```python
from build123d import *

# Parameters (mm, degrees)
CROQUIS1_W                        = 55
CROQUIS1_H                        = 58
CROQUIS1_R                        = 2.2
SALIENTE_EXTRUIR1_DEPTH           = 6
CROQUIS2_R                        = 4.5
CORTAR_EXTRUIR1_DEPTH             = 3
REDONDEO1_R                       = 1
CROQUIS3_W                        = 55
CROQUIS3_H                        = 40
SALIENTE_EXTRUIR2_DEPTH           = 5
CROQUIS4_W                        = 55
CROQUIS4_H                        = 10
SALIENTE_EXTRUIR3_DEPTH           = 14
CORTAR_EXTRUIR2_DEPTH             = 71.577971067
CORTAR_EXTRUIR2_DEPTH_BACK        = 71.577971067
CROQUIS5_R                        = 3.3
CORTAR_EXTRUIR3_REACH             = 127.623
SALIENTE_EXTRUIR4_REACH           = 69.47
CORTAR_EXTRUIR4_DEPTH             = 118.48297749
CORTAR_EXTRUIR5_REACH             = 99.372
CORTAR_EXTRUIR5_DIRECTION_2_REACH = 99.372
CROQUIS10_W                       = 21
CROQUIS10_H                       = 42
CORTAR_EXTRUIR6_DEPTH             = 98.371710471
CROQUIS11_W                       = 33
CROQUIS11_H                       = 63.666666667
CORTAR_EXTRUIR7_DEPTH             = 5.5
CROQUIS12_R                       = 2
CORTAR_EXTRUIR8_DEPTH             = 97.106711524
CORTAR_EXTRUIR9_DEPTH             = 3
CHAFL_N1_SIZE                     = 2
CROQUIS14_R                       = 1.75
CORTAR_EXTRUIR10_DEPTH            = 98.371710471
CORTAR_EXTRUIR11_DEPTH            = 2.5
REDONDEO2_R                       = 5


with BuildPart() as part:
    # Croquis1 → Saliente-Extruir1 (new body)
    with BuildSketch(Plane(origin=(0, 0, 0), x_dir=(1, 0, 0), z_dir=(0, 1, 0))):
        Rectangle(CROQUIS1_W, CROQUIS1_H)
        with Locations(Location((-12.5, 13.181818182, 0), (0, 0, 270))):
            Circle(CROQUIS1_R, mode=Mode.SUBTRACT)
        with Locations(Location((12.5, 13.181818182, 0), (0, 0, 270))):
            Circle(CROQUIS1_R, mode=Mode.SUBTRACT)
        with Locations(Location((-12.5, -13.181818182, 0), (0, 0, 270))):
            Circle(CROQUIS1_R, mode=Mode.SUBTRACT)
        with Locations(Location((12.5, -13.181818182, 0), (0, 0, 270))):
            Circle(CROQUIS1_R, mode=Mode.SUBTRACT)
    extrude(amount=SALIENTE_EXTRUIR1_DEPTH)

    # Croquis2 → Cortar-Extruir1 (cut)
    with BuildSketch(Plane(origin=(0, 6, 0), x_dir=(1, 0, 0), z_dir=(0, 1, 0))):
        with Locations(Location((-12.5, 13.181818182, 0), (0, 0, 270))):
            Circle(CROQUIS2_R)
        with Locations(Location((12.5, 13.181818182, 0), (0, 0, 270))):
            Circle(CROQUIS2_R)
        with Locations(Location((-12.5, -13.181818182, 0), (0, 0, 270))):
            Circle(CROQUIS2_R)
        with Locations(Location((12.5, -13.181818182, 0), (0, 0, 270))):
            Circle(CROQUIS2_R)
    extrude(amount=-CORTAR_EXTRUIR1_DEPTH, mode=Mode.SUBTRACT)

    # Redondeo1
    redondeo1_edges = [part.edges().sort_by_distance(p)[0] for p in [
        (12.5, 6, -17.681818182),
        (-12.5, 6, 8.681818182),
        (12.5, 6, 8.681818182),
        (-12.5, 6, -17.681818182),
    ]]
    fillet(redondeo1_edges, radius=REDONDEO1_R)

    # Croquis3 → Saliente-Extruir2 (add)
    with BuildSketch(Plane(origin=(0, 6, 0), x_dir=(1, 0, 0), z_dir=(0, 1, 0))):
        with Locations((0, 40)):
            Rectangle(CROQUIS3_W, CROQUIS3_H)
        with Locations((0, -40)):
            Rectangle(CROQUIS3_W, CROQUIS3_H)
    extrude(amount=SALIENTE_EXTRUIR2_DEPTH)

    # Croquis4 → Saliente-Extruir3 (add)
    with BuildSketch(Plane(origin=(0, 11, 0), x_dir=(1, 0, 0), z_dir=(0, 1, 0))):
        with Locations((0, 55)):
            Rectangle(CROQUIS4_W, CROQUIS4_H)
        with Locations((0, -55)):
            Rectangle(CROQUIS4_W, CROQUIS4_H)
    extrude(amount=SALIENTE_EXTRUIR3_DEPTH)

    # Croquis5 → Cortar-Extruir2 (cut, two sides: drawn at the far end of the back side and taken through both)
    with BuildSketch(Plane.XY.offset(-CORTAR_EXTRUIR2_DEPTH_BACK)):
        with Locations((-20, 18)):
            Circle(CROQUIS5_R)
        with Locations((20, 18)):
            Circle(CROQUIS5_R)
    extrude(amount=CORTAR_EXTRUIR2_DEPTH + CORTAR_EXTRUIR2_DEPTH_BACK, mode=Mode.SUBTRACT)

    # Croquis6 → Cortar-Extruir3 (cut, up to next)
    with BuildSketch(Plane(origin=(0, 0, -60), x_dir=(-1, 0, 0), z_dir=(0, 0, -1)), mode=Mode.PRIVATE) as cortar_extruir3_sk1:
        with BuildLine():
            Line((27.5, 23.5), (20, 23.5))
            ThreePointArc((20, 23.5), (14.5, 18), (20, 12.5))
            Line((20, 12.5), (27.5, 12.5))
            Line((27.5, 12.5), (27.5, 23.5))
        make_face()
    cortar_extruir3_tool1 = extrude(cortar_extruir3_sk1.sketch, amount=-CORTAR_EXTRUIR3_REACH, mode=Mode.PRIVATE) & part.part
    add(cortar_extruir3_tool1.solids().sort_by_distance((-21.526408, 18, -60))[0], mode=Mode.SUBTRACT)

    # Saliente-Extruir4: up to this face of the body (flat: up to its plane)
    saliente_extruir4_end = Plane(part.part.faces().sort_by_distance((0, 0, 0))[0])
    # Croquis7 → Saliente-Extruir4 (add, up to the picked face)
    with BuildSketch(Plane(origin=(0, 11, 0), x_dir=(1, 0, 0), z_dir=(0, 1, 0)), mode=Mode.PRIVATE) as saliente_extruir4_sk1:
        Polygon((-72.5, 30), (-72.5, -30), (-27.5, -50), (-27.5, 50), align=None)
    saliente_extruir4_tool1 = split(extrude(saliente_extruir4_sk1.sketch, amount=-SALIENTE_EXTRUIR4_REACH, mode=Mode.PRIVATE), bisect_by=saliente_extruir4_end, keep=Keep.BOTH, mode=Mode.PRIVATE)
    add(saliente_extruir4_tool1.solids().sort_by(Axis((-48.125, 11, 0), (0, -1, 0)))[0])

    # Croquis8 → Cortar-Extruir4 (cut, through all)
    with BuildSketch(Plane(origin=(0, 0, -29), x_dir=(-1, 0, 0), z_dir=(0, 0, -1))):
        Polygon((27.5, 6), (47.5, 0), (27.5, 0), align=None)
    cortar_extruir4 = extrude(amount=CORTAR_EXTRUIR4_DEPTH, mode=Mode.SUBTRACT)

    # Simetría1: Cortar-Extruir4 across plane
    add(cortar_extruir4.mirror(Plane.XY), mode=Mode.SUBTRACT)

    # Cortar-Extruir5: up to this face of the body (flat: up to its plane)
    cortar_extruir5_end = Plane(part.part.faces().sort_by_distance((0, 8.5, -20))[0])
    # Croquis9 → Cortar-Extruir5 (cut, up to the picked face)
    with BuildSketch(Plane.XY, mode=Mode.PRIVATE) as cortar_extruir5_sk1:
        Polygon((-27.5, 6), (-50, 11), (-27.5, 11), align=None)
    cortar_extruir5_tool1 = split(extrude(cortar_extruir5_sk1.sketch, amount=-CORTAR_EXTRUIR5_REACH, mode=Mode.PRIVATE), bisect_by=cortar_extruir5_end, keep=Keep.BOTH, mode=Mode.PRIVATE)
    add(cortar_extruir5_tool1.solids().sort_by(Axis((-35, 9.333333, 0), (0, 0, -1)))[0], mode=Mode.SUBTRACT)

    # Cortar-Extruir5 direction 2: up to this face of the body (flat: up to its plane)
    cortar_extruir5_direction_2_end = Plane(part.part.faces().sort_by_distance((0, 8.5, 20))[0])
    # Croquis9 → Cortar-Extruir5 direction 2 (cut, up to the picked face)
    with BuildSketch(Plane.XY, mode=Mode.PRIVATE) as cortar_extruir5_direction_2_sk1:
        Polygon((-27.5, 6), (-50, 11), (-27.5, 11), align=None)
    cortar_extruir5_direction_2_tool1 = split(extrude(cortar_extruir5_direction_2_sk1.sketch, amount=CORTAR_EXTRUIR5_DIRECTION_2_REACH, mode=Mode.PRIVATE), bisect_by=cortar_extruir5_direction_2_end, keep=Keep.BOTH, mode=Mode.PRIVATE)
    add(cortar_extruir5_direction_2_tool1.solids().sort_by(Axis((-35, 9.333333, 0), (0, 0, 1)))[0], mode=Mode.SUBTRACT)

    # Croquis10 → Cortar-Extruir6 (cut, through all)
    with BuildSketch(Plane.XZ):
        with Locations((-50, 10)):
            Rectangle(CROQUIS10_W, CROQUIS10_H)
    extrude(amount=-CORTAR_EXTRUIR6_DEPTH, mode=Mode.SUBTRACT)

    # Croquis11 → Cortar-Extruir7 (cut)
    with BuildSketch(Plane.XZ):
        with Locations((-56, 12.833333334)):
            Rectangle(CROQUIS11_W, CROQUIS11_H)
    extrude(amount=-CORTAR_EXTRUIR7_DEPTH, mode=Mode.SUBTRACT)

    # Croquis12 → Cortar-Extruir8 (cut, through all)
    with BuildSketch(Plane.XZ.offset(-5.5)):
        with Locations(Location((-45, 34, 0), (0, 0, 270))):
            Circle(CROQUIS12_R)
        with Locations(Location((-55, 34, 0), (0, 0, 270))):
            Circle(CROQUIS12_R)
        with Locations(Location((-55, -13.5, 0), (0, 0, 270))):
            Circle(CROQUIS12_R)
        with Locations((-45, -13.5)):
            Circle(CROQUIS12_R)
    extrude(amount=-CORTAR_EXTRUIR8_DEPTH, mode=Mode.SUBTRACT)

    # Croquis13 → Cortar-Extruir9 (cut)
    with BuildSketch(Plane(origin=(0, 11, 0), x_dir=(1, 0, 0), z_dir=(0, 1, 0))):
        Polygon((-72.5, 20), (-39.5, 20), (-39.5, -39), (-52.25, -39), (-72.5, -30), align=None)
    extrude(amount=-CORTAR_EXTRUIR9_DEPTH, mode=Mode.SUBTRACT)

    # Chaflán1
    chafl_n1_edges = [part.edges().sort_by_distance(p)[0] for p in [
        (-6, 0, 29),
        (-56, 0, -19),
        (-10, 0, -29),
        (-22.5, 11, -20),
        (-6, 11, 20),
    ]]
    chamfer(chafl_n1_edges, length=CHAFL_N1_SIZE)

    # Croquis14 → Cortar-Extruir10 (cut, through all)
    with BuildSketch(Plane(origin=(0, 25, 0), x_dir=(1, 0, 0), z_dir=(0, 1, 0))):
        with Locations(Location((0, 55, 0), (0, 0, 270))):
            Circle(CROQUIS14_R)
        with Locations(Location((0, -55, 0), (0, 0, 270))):
            Circle(CROQUIS14_R)
    extrude(amount=-CORTAR_EXTRUIR10_DEPTH, mode=Mode.SUBTRACT)

    # Croquis15 → Cortar-Extruir11 (cut)
    with BuildSketch(Plane.XZ.offset(-6)):
        Polygon((3.810511777, 55), (1.905255888, 58.3), (-1.905255888, 58.3), (-3.810511777, 55), (-1.905255888, 51.7), (1.905255888, 51.7), align=None)
        Polygon((1.905255888, -51.7), (3.810511777, -55), (1.905255888, -58.3), (-1.905255888, -58.3), (-3.810511777, -55), (-1.905255888, -51.7), align=None)
    extrude(amount=-CORTAR_EXTRUIR11_DEPTH, mode=Mode.SUBTRACT)

    # Redondeo2
    redondeo2_edges = [part.edges().sort_by_distance(p)[0] for p in [
        (-72.5, 5.5, -30),
        (-72.5, 6.75, 30),
    ]]
    fillet(redondeo2_edges, radius=REDONDEO2_R)


solid = part.part
```
Here's how the part is built. I have some questions about the finished solid (model axes, mm). A direction names the side the tool comes from. Coordinates: 2 decimals unless noted, no trailing zeros. Loops run counter-clockwise (first coordinate to the right, second up) from the corner with the lowest first, then second, coordinate; pieces in that order, holes last. Notation, with made-up numbers: (-25.75, 4.5) -> (-19.75, 4.5) arc R16 ccw to (-19.75, 28.5) -> close; hole circle Ø2 at (14, -15). An arc over 180 degrees is marked (long way). Return JSON: item names as keys, results as strings.
1) If we section it at C-C, the plane x = 12.5: Count the separate pieces of the cut face and the enclosed holes in it, then the cut area to 3 significant figures.
Results below:
{"separate pieces": "3", "enclosed holes": "0", "area": "939 mm²"}
2) For faces 4 (the face through (-24, 12.5, -55)), 5 (the face through (13.85, 4.01, -8.89)), 6 (the face through (2.845, 7.232, -53.327)), 7 (the face through (-64, 5.5, 6)), 8 (the face through (6, 18, -50)), which set-ups out of +Z, -Z, +X, -X, +Y, -Y let a thin tool reach every point of the face, with its end or its side?
Results below:
{"face 4": "-Z, -X", "face 5": "+Y", "face 6": "-Y", "face 7": "+Z, -X, -Y", "face 8": "+X, -X, +Y"}
3) Thinking about a two-plate mould opening in Y: for faces 1 (the face through (-14.5, 18.1, -55.1)), 2 (the face through (-12, 0, 1)), 3 (the face through (-2.845, 7.232, -56.673)), which applies, +Y half, -Y half, draft (parallel to the pull), parting line (faces both ways), or undercut?
Results below:
{"face 1": "undercut", "face 2": "-Y half", "face 3": "draft"}
4) If we section it at A-A, the plane y = 18: Write out the boundary of the cut face in (x, z).
Results below:
{"outline": "(-27.5, 50) -> (-23.3, 50) -> (-23.3, 60) -> (-27.5, 60) -> close; (-16.7, 50) -> (16.7, 50) -> (16.7, 60) -> (-16.7, 60) -> close; (-14.5, -60) -> (16.7, -60) -> (16.7, -50) -> (-14.5, -50) -> close; (23.3, -60) -> (27.5, -60) -> (27.5, -50) -> (23.3, -50) -> close; (23.3, 50) -> (27.5, 50) -> (27.5, 60) -> (23.3, 60) -> close; hole circle Ø3.5 at (0, -55); hole circle Ø3.5 at (0, 55)"}
5) I need wall thicknesses on line 1 (X direction, y = 18, z = 55.25); line 2 (Y direction, x = 23, z = -42.5); line 3 (Z direction, x = 18, y = 10). Which ranges of each line are inside material? Lowest first, please. Write a range as from..to.
Results below:
{"line 1": "-27.5..-23.3, -16.7..-1.73, 1.73..16.7, 23.3..27.5", "line 2": "6..11", "line 3": "-60..-21, 21..60"}
6) Will these pins go through, and if not, where does the flat tip stop? pin 1 (10 mm diameter, centred on x = 13.5, z = 12, fed in from +Y); pin 2 (2 mm diameter, centred on y = 10, z = -53, fed in from -X); pin 3 (14 mm diameter, centred on x = -7.5, z = 41, fed in from +Y); pin 4 (5.5 mm diameter, centred on x = 20, y = 18, fed in from +Z).
Results below:
{"pin 1": "y = 6", "pin 2": "x = -27.5", "pin 3": "y = 11", "pin 4": "through"}
7) If we section it at B-B, the plane x = -45: Write out the boundary of the cut face in (y, z), then the cut area to 3 significant figures.
Results below:
{"outline": "(0, -27) -> (0.75, -27.75) -> (0.75, -42.22) -> (11, -42.22) -> (11, -22) -> (9, -20) -> (8, -20) -> (8, -15.5) -> (5.5, -15.5) -> (5.5, -19) -> (2, -19) -> (0, -21) -> close; (5.5, -11.5) -> (8, -11.5) -> (8, -11) -> (5.5, -11) -> close; (5.5, 31) -> (8, 31) -> (8, 32) -> (5.5, 32) -> close; (5.5, 36) -> (8, 36) -> (8, 39) -> (11, 39) -> (11, 42.22) -> (5.5, 42.22) -> close", "area": "275 mm²"}
